Autodesk Inventor part; units mm, degrees
ref_plane "YZ Plane" through (0, 0, 0) normal (1, 0, 0) x (0, 1, 0)
ref_plane "XZ Plane" through (0, 0, 0) normal (0, 1, 0) x (-1, 0, 0)
ref_plane "XY Plane" through (0, 0, 0) normal (0, 0, 1) x (1, 0, 0)
sketch "Skizze1" plane through (0, 0, 0) normal (0, 1, 0) x (-1, 0, 0)
  line L0 (0, 0) -> (255.6, 0)
  line L1 (255.6, 0) -> (255.6, -287.6)
  line L2 (255.6, -287.6) -> (0, -287.6)
  line L3 (0, -287.6) -> (0, 0)
  dimension "d0" = 287.6
  dimension "d1" = 255.6
extrude "Extrusion1" add sketch "Skizze1" along normal blind 10
sketch "Skizze4" plane through (0, 10, 0) normal (0, 1, 0) x (1, 0, 0)
  line L0 (-25, 25) -> (-33.2, 25)
  line L1 (-33.2, 25) -> (-33.2, 37.2)
  line L2 (-33.2, 37.2) -> (-25, 37.2)
  line L3 (-25, 37.2) -> (-25, 25)
  line L4 (-109.6, 25) -> (-117.8, 25)
  line L5 (-117.8, 25) -> (-117.8, 38.7)
  line L6 (-117.8, 38.7) -> (-109.6, 38.7)
  line L7 (-109.6, 38.7) -> (-109.6, 25)
  line L8 (-137.8, 25) -> (-146, 25)
  line L9 (-146, 25) -> (-146, 39.2)
  line L10 (-146, 39.2) -> (-137.8, 39.2)
  line L11 (-137.8, 39.2) -> (-137.8, 25)
  line L12 (-166, 39.7) -> (-166, 25)
  line L13 (-222.4, 25) -> (-230.6, 25)
  line L14 (-230.6, 25) -> (-230.6, 40.7)
  line L15 (-25, 57.2) -> (-33.7, 57.2)
  line L16 (-33.7, 57.2) -> (-33.7, 69.4)
  line L17 (-33.7, 69.4) -> (-25, 69.4)
  line L18 (-25, 69.4) -> (-25, 57.2)
  line L19 (-25, 89.4) -> (-34.2, 89.4)
  line L20 (-34.2, 89.4) -> (-34.2, 101.6)
  line L21 (-34.2, 101.6) -> (-25, 101.6)
  line L22 (-25, 101.6) -> (-25, 89.4)
  line L23 (-25, 121.6) -> (-34.7, 121.6)
  line L24 (-34.7, 121.6) -> (-34.7, 133.8)
  line L25 (-34.7, 133.8) -> (-25, 133.8)
  line L26 (-25, 133.8) -> (-25, 121.6)
  line L27 (-25, 153.8) -> (-35.2, 153.8)
  line L28 (-35.2, 153.8) -> (-35.2, 166)
  line L29 (-35.2, 166) -> (-25, 166)
  line L30 (-25, 166) -> (-25, 153.8)
  line L31 (-25, 186) -> (-35.7, 186)
  line L32 (-35.7, 186) -> (-35.7, 198.2)
  line L33 (-35.7, 198.2) -> (-25, 198.2)
  line L34 (-25, 198.2) -> (-25, 186)
  line L35 (-25, 230.4) -> (-25, 218.2)
  line L36 (-222.4, 25) -> (-222.4, 38.5)
  line L37 (-222.4, 38.5) -> (-222.4, 40.7)
  line L38 (-230.6, 40.7) -> (-222.4, 40.7)
  line L39 (-25, 218.2) -> (-36.2, 218.2)
  line L40 (-36.2, 218.2) -> (-36.2, 230.4)
  line L41 (-36.2, 230.4) -> (-25, 230.4)
  line L42 (-25, 250.4) -> (-25, 262.6)
  line L43 (-25, 262.6) -> (-36.7, 262.6)
  line L44 (-36.7, 262.6) -> (-36.7, 250.4)
  line L45 (-36.7, 250.4) -> (-25, 250.4)
  line L46 (-53.2, 25) -> (-61.4, 25)
  line L47 (-61.4, 25) -> (-61.4, 37.7)
  line L48 (-61.4, 37.7) -> (-53.2, 37.7)
  line L49 (-53.2, 37.7) -> (-53.2, 25)
  line L50 (-89.6, 25) -> (-89.6, 37.7)
  line L51 (-89.6, 37.7) -> (-89.6, 38.2)
  line L52 (0, 0) -> (0, 287.6)
  line L53 (-255.6, 0) -> (0, 0)
  line L54 (-81.4, 69.9) -> (-90.1, 69.9)
  line L55 (-90.1, 69.9) -> (-90.1, 57.2)
  line L56 (-90.1, 57.2) -> (-81.4, 57.2)
  line L57 (-81.4, 102.6) -> (-90.6, 102.6)
  line L58 (-90.6, 102.6) -> (-90.6, 89.4)
  line L59 (-90.6, 89.4) -> (-81.4, 89.4)
  line L60 (-81.4, 121.6) -> (-81.4, 135.3)
  line L61 (-81.4, 135.3) -> (-91.1, 135.3)
  line L62 (-91.1, 135.3) -> (-91.1, 121.6)
  line L63 (-91.1, 121.6) -> (-81.4, 121.6)
  line L64 (-81.4, 153.8) -> (-81.4, 168)
  line L65 (-81.4, 168) -> (-91.6, 168)
  line L66 (-91.6, 168) -> (-91.6, 153.8)
  line L67 (-91.6, 153.8) -> (-81.4, 153.8)
  line L68 (-81.4, 186) -> (-81.4, 200.7)
  line L69 (-81.4, 200.7) -> (-92.1, 200.7)
  line L70 (-92.1, 200.7) -> (-92.1, 186)
  line L71 (-92.1, 186) -> (-81.4, 186)
  line L72 (-81.4, 218.2) -> (-81.4, 233.4)
  line L73 (-81.4, 233.4) -> (-92.6, 233.4)
  line L74 (-92.6, 233.4) -> (-92.6, 218.2)
  line L75 (-92.6, 218.2) -> (-81.4, 218.2)
  line L76 (-81.4, 250.4) -> (-81.4, 266.1)
  line L77 (-81.4, 266.1) -> (-93.1, 266.1)
  line L78 (-93.1, 266.1) -> (-93.1, 250.4)
  line L79 (-93.1, 250.4) -> (-81.4, 250.4)
  line L80 (-194.2, 25) -> (-202.4, 25)
  line L81 (-202.4, 25) -> (-202.4, 40.2)
  line L82 (-202.4, 40.2) -> (-194.2, 40.2)
  line L83 (-194.2, 40.2) -> (-194.2, 25)
  line L84 (-166, 25) -> (-174.2, 25)
  line L85 (-166, 39.7) -> (-174.2, 39.7)
  line L86 (-174.2, 39.7) -> (-174.2, 25)
  line L87 (-166, 25) -> (-174.2, 25)
  line L88 (-81.4, 25) -> (-89.6, 25)
  line L89 (-81.4, 25) -> (-81.4, 38.2)
  line L90 (-81.4, 38.2) -> (-89.6, 38.2)
  line L91 (-202.4, 25) -> (-194.2, 25)
  line L92 (-174.2, 25) -> (-166, 25)
  line L93 (-146, 25) -> (-137.8, 25)
  line L94 (-137.8, 25) -> (-146, 25)
  line L95 (-109.6, 25) -> (-117.8, 25)
  line L96 (-81.4, 25) -> (-89.6, 25)
  line L97 (-25, 25) -> (-33.2, 25)
  line L98 (-53.2, 25) -> (-61.4, 25)
  line L99 (-166, 25) -> (-174.2, 25)
  line L100 (-194.2, 25) -> (-202.4, 25)
  line L101 (-222.4, 25) -> (-230.6, 25)
  line L102 (-25, 57.2) -> (-33.7, 57.2)
  line L103 (-81.4, 57.2) -> (-90.1, 57.2)
  line L104 (-25, 89.4) -> (-34.2, 89.4)
  line L105 (-81.4, 89.4) -> (-90.6, 89.4)
  line L106 (-25, 121.6) -> (-34.7, 121.6)
  line L107 (-81.4, 121.6) -> (-91.1, 121.6)
  line L108 (-25, 153.8) -> (-35.2, 153.8)
  line L109 (-81.4, 153.8) -> (-91.6, 153.8)
  line L110 (-25, 186) -> (-35.7, 186)
  line L111 (-81.4, 186) -> (-92.1, 186)
  line L112 (-25, 218.2) -> (-36.2, 218.2)
  line L113 (-81.4, 218.2) -> (-92.6, 218.2)
  line L114 (-25, 250.4) -> (-36.7, 250.4)
  line L115 (-81.4, 250.4) -> (-93.1, 250.4)
  line L116 (-81.4, 26.1) -> (-81.4, 294.0046)
  line L117 (-81.4, 69.9) -> (-81.4, 47.2)
  line L118 (-90.1, 57.2) -> (-90.1, 69.9)
  line L119 (-81.4, 89.4) -> (-81.4, 102.6)
  line L120 (-90.6, 102.6) -> (-90.6, 89.4)
  line L121 (-25, 25) -> (-25, 285.2671)
  line L122 (-25, 25) -> (-258.6914, 25)
  line L123 (0, 287.6) -> (-255.6, 287.6)
  line L124 (-255.6, 287.6) -> (-255.6, 0)
  point P0 (-29.6, 89.4)
  point P1 (-29.35, 69.4)
  point P2 (-29.85, 121.6)
  point P3 (-29.6, 101.6)
  point P4 (-30.1, 153.8)
  point P5 (-29.85, 133.8)
  point P6 (-30.35, 186)
  point P7 (-30.1, 166)
  point P8 (-30.6, 218.2)
  point P9 (-30.35, 198.2)
  point P10 (-30.85, 250.4)
  point P11 (-30.6, 230.4)
  point P12 (-81.4, 25)
  point P13 (-53.2, 31.35)
  point P14 (-61.4, 31.35)
  point P15 (-109.6, 31.85)
  point P16 (-137.8, 32.1)
  point P17 (-117.8, 31.85)
  point P18 (-166, 27.1)
  point P19 (-146, 32.1)
  point P20 (-169.2, 27.6)
  point P21 (-222.4, 31.75)
  point P22 (-25, 31.1)
  point P23 (-29.1, 25)
  point P24 (-29.35, 57.2)
  point P25 (-85.75, 57.2)
  point P26 (-86.25, 121.6)
  point P27 (-141.9, 25)
  point P28 (-86.5, 153.8)
  point P29 (-86.75, 186)
  point P30 (-87, 218.2)
  point P31 (-81.4, 225.8)
  point P32 (-81.4, 258.25)
  point P33 (-226.5, 40.7)
  point P34 (-86, 102.6)
  point P35 (-86.25, 135.3)
  point P36 (-86.75, 200.7)
  point P37 (-87.25, 250.4)
  point P38 (-87, 233.4)
  point P39 (-86, 89.4)
  point P40 (-85.75, 69.9)
  point P41 (-86.5, 168)
  point P42 (-33.7, 63.3)
  point P43 (-80, 91)
  point P44 (-34.2, 95.5)
  point P45 (-81.4, 128.45)
  point P46 (-34.7, 127.7)
  point P47 (-81.4, 160.9)
  point P48 (-35.2, 159.9)
  point P49 (-81.4, 193.35)
  point P50 (-35.7, 192.1)
  point P51 (-36.2, 224.3)
  point P52 (-36.7, 256.5)
  point P53 (-81.4, 58.55)
  point P54 (-76, 52.7)
  point P55 (-76, 65.4)
  point P56 (-25, 256.5)
  point P57 (-57.3, 25)
  point P58 (-29.6, 89.4)
  point P59 (-86, 89.4)
  point P60 (-87, 218.2)
  point P61 (-30.6, 218.2)
  point P62 (-87.25, 250.4)
  point P63 (-30.85, 250.4)
  point P64 (-85.75, 57.2)
  point P65 (-85.5, 38.2)
  point P66 (-29.35, 57.2)
  point P67 (-30.35, 186)
  point P68 (-87.25, 266.1)
  point P69 (-30.85, 262.6)
  point P70 (-230.6, 32.85)
  point P71 (-81.4, 31.6)
  point P72 (-226.5, 25)
  dimension "d10" = 8.2
  dimension "d11" = 12.2
  dimension "d17" = 12.2
  dimension "d18" = 9.2
  dimension "d19" = 12.2
  dimension "d20" = 9.7
  dimension "d21" = 12.2
  dimension "d22" = 10.2
  dimension "d23" = 12.2
  dimension "d24" = 10.7
  dimension "d25" = 12.2
  dimension "d27" = 12.2
  dimension "d29" = 13.7
  dimension "d30" = 14.2
  dimension "d32" = 14.7
  dimension "d53" = 11.2
  dimension "d60" = 12.2
  dimension "d61" = 11.7
  dimension "d64" = 12.7
  dimension "d65" = 8.2
  dimension "d79" = 12.7
  dimension "d80" = 13.2
  dimension "d81" = 9.2
  dimension "d82" = 13.7
  dimension "d83" = 9.7
  dimension "d84" = 14.2
  dimension "d85" = 10.2
  dimension "d86" = 14.7
  dimension "d87" = 10.7
  dimension "d88" = 15.2
  dimension "d89" = 11.2
  dimension "d90" = 15.7
  dimension "d91" = 11.7
  dimension "d149" = 15.7
  dimension "d152" = 8.2
  dimension "d153" = 8.2
  dimension "d155" = 20
  dimension "d156" = 8.2
  dimension "d159" = 20
  dimension "d160" = 20
  dimension "d162" = 20
  dimension "d163" = 20
  dimension "d164" = 20
  dimension "d165" = 20
  dimension "d166" = 20
  dimension "d167" = 20
  dimension "d168" = 20
  dimension "d169" = 20
  dimension "d187" = 19
  dimension "d188" = 18.5
  dimension "d189" = 18
  dimension "d191" = 17.5
  dimension "d197" = 8.2
  dimension "d198" = 15.2
  dimension "d199" = 20
  dimension "d200" = 8.2
  dimension "d201" = 20
  dimension "d203" = 8.2
  dimension "d205" = 13.2
  dimension "d207" = 8.7
  dimension "d209" = 45.8
  dimension "d219" = 8.7
  dimension "d239" = 0
  dimension "d240" = 0
extrude "Extrusion4" cut sketch "Skizze4" against normal blind 30 contours L88 L50 L51 L90 L89 | L46 L47 L48 L49 | L45 L44 L43 L42 | L39 L40 L41 L35 | L31 L32 L33 L34 | L27 L28 L29 L30 | L23 L24 L25 L26 | L19 L20 L21 L22 | L15 L16 L17 L18 | L0 L1 L2 L3 | L4 L5 L6 L7 | L8 L9 L10 L11 | L56 L55 L54 L116 | L84 L86 L85 L12 | L59 L58 L57 L116 | L80 L81 L82 L83 | L63 L62 L61 L60 | L13 L14 L38 L37 L36 | L67 L66 L65 L64 | L71 L70 L69 L68 | L75 L74 L73 L72 | L76 L79 L78 L77
sketch "Skizze5" plane through (0, 10, 0) normal (0, 1, 0) x (1, 0, 0)
  circle A0 centre (-215.6, 100) radius 2.5
  circle A1 centre (-215.6, 204) radius 2.5
  line L0 (-255.6, 0) -> (0, 0)
  line L1 (-255.6, 287.6) -> (-255.6, 0)
  circle A2 centre (-171.6, 100) radius 2.5
  circle A3 centre (-171.6, 204) radius 2.5
  line L2 (-171.6, 100) -> (-215.6, 100)
  line L3 (-215.6, 100) -> (-215.6, 204)
  line L4 (-215.6, 204) -> (-171.6, 204)
  line L5 (-171.6, 204) -> (-171.6, 100)
  dimension "d110" = 5
  dimension "d116" = 5
  dimension "d119" = 100
  dimension "d224" = 5
  dimension "d225" = 5
  dimension "d230" = 104
  dimension "d231" = 44
  dimension "d233" = 40
  dimension "d234" = 0
extrude "Extrusion5" cut sketch "Skizze5" against normal blind 30 contours L2 L3 A0 | A0 L3 L2 | L2 L5 A2 | A2 L5 L2 | L3 L4 A1 | A1 L4 L3 | L5 L4 A3 | A3 L4 L5
sketch "Skizze6" plane through (0, 0, 0) normal (0, -1, 0) x (1, 0, 0)
  line L0 (-255.6, -287.6) -> (-255.6, 0)
  line L1 (-255.6, 0) -> (0, 0)
  line L2 (0, 0) -> (0, -287.6)
  line L3 (0, -287.6) -> (-255.6, -287.6)
  point P0 (-240.6, -15)
  point P1 (-240.6, -272.6)
  point P2 (-15, -272.6)
  point P3 (-15, -15)
  dimension "d265" = 15
  dimension "d266" = 15
  dimension "d267" = 15
  dimension "d268" = 15
  dimension "d269" = 15
  dimension "d270" = 15
  dimension "d271" = 15
  dimension "d272" = 15
hole "Bohrung1" at (-240.6, 0, -15) at (-240.6, 0, -272.6) at (-15, 0, -272.6) at (-15, 0, -15) direction (0, 1, 0) diameter 7 depth 10
properties part number "Board_Maria_3D-Druck"
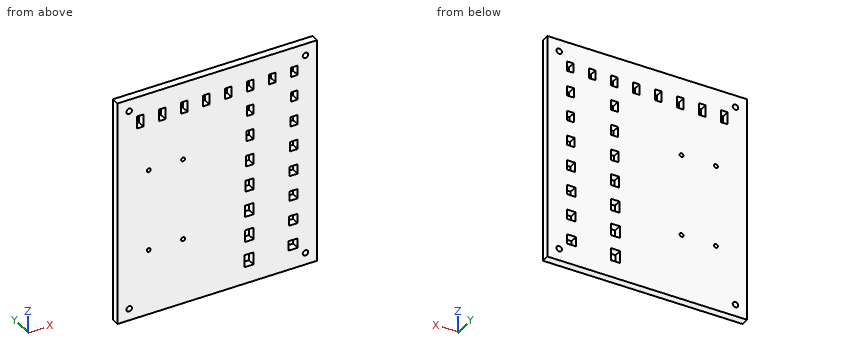
Model file for the job. Use its own axes, mm. Give positions to 0.01 mm unless a question says otherwise; leave off trailing zeros. Loops run counter-clockwise (first coordinate to the right, second up) from the corner with the lowest first, then second, coordinate; pieces in that order, holes last. Notation, with made-up numbers: (4.5, 68.25) -> (43.5, 68.25) arc R9 ccw to (43.5, 79.25) -> close; hole circle Ø2 at (48, 43.5). An arc over 180 degrees is marked (long way). Write each question's results on one line, items separated by ' | '.
(1) Flat gauge pin, fed straight in: pin 1 Ø3 at (x, z) = (-171.6, -100) entering from +Y. Where does the tip first touch, or does it go through?
Geometry results:
pin 1: passes through
(2) Cut at A-A on z = -129.5. List the corners of the cut face in (x, y), and give its area (3 significant figures).
Geometry results:
outline: (-255.6, 0) -> (-91.1, 0) -> (-91.1, 10) -> (-255.6, 10) -> close; (-81.4, 0) -> (-34.7, 0) -> (-34.7, 10) -> (-81.4, 10) -> close; (-25, 0) -> (0, 0) -> (0, 10) -> (-25, 10) -> close | area: 2,360 mm²
(3) Cut at B-B on x = -15. List the corners of the cut face in (y, z), and give its area (3 significant figures).
Geometry results:
outline: (0, -287.6) -> (10, -287.6) -> (10, -276.1) -> (0, -276.1) -> close; (0, -269.1) -> (10, -269.1) -> (10, -18.5) -> (0, -18.5) -> close; (0, -11.5) -> (10, -11.5) -> (10, 0) -> (0, 0) -> close | area: 2,740 mm²
(4) Cut at C-C on y = 2. Give the number of separate pieces and of enclosed holes in the cut face, and give its area (3 significant figures).
Geometry results:
separate pieces: 1 | enclosed holes: 30 | area: 70,500 mm²
(5) Probe line 1 along Z through (x, y) = (-15, 4.75); line 2 along X through (y, z) = (6.5, -158); line 3 along Z through (x, y) = (-215, 1.75). List the from-to ranges inside material, lowest first.
Geometry results:
line 1: z = -287.6 to -276.1, -269.1 to -18.5, -11.5 to 0 | line 2: x = -255.6 to -91.6, -81.4 to -35.2, -25 to 0 | line 3: z = -287.6 to -206.43, -201.57 to -102.43, -97.57 to 0
